Read the model definition and answer for the solid it produces. Units are mm, in the model's axes. A direction names the side the tool comes from. Give positions to 0.01 mm unless a question says otherwise; leave off trailing zeros. Order: outer loops, then holes, each group sorted by start corner. A loop starts at its lowest first (then second) coordinate and runs counter-clockwise, first axis right, second up. Notation, with made-up numbers: (-37.5, -8) -> (6.5, -8) arc R11 ccw to (6.5, -1) -> close; hole circle Ø1 at (-22.75, 8). An arc over 180 degrees is marked (long way). Answer as CSV lines item,"result". Start each with the question number.
1) For faces 1 (the face through (-3.905, 0.986, -0.867)), 2 (the face through (-10, 7, 13)), determine the directions among +Z, -Z, +X, -X, +Y, -Y from which every point of the face is accessible in a straight line to the end or side of a thin tool.
2) The mould has two halves that part along X. Classify faces 3 (the face through (0, 1, -12)), 4 (the face through (11, 15, 18)), 5 (the face through (2, 2, 4)), 6 (the face through (-12, 6, 12)): +X half, -X half, draft (parallel to the pull), parting line (faces both ways), or undercut.
3) Find section C-C (y = 13.75). Determine the outline of the cut face in (x, z), and give its area (3 significant figures).
4) Find section D-D (y = 1). Determine the outline of the cut face in (x, z).
5) Find section B-B (z = 16). Determine the outline of the cut face in (x, y).
6) Straight lines are drawn through the part: L1, parallel to X at y = 0.95, z = 0; L2, parallel to X at y = 4.5, z = 11; L3, parallel to Y at x = 9, z = 15. For each, find the intervals that lie inside material, in ascending order. Write a range as from..to.
7) Flat-ended cylindrical pins translate along their axes: pin 1 Ø2 at (x, z) = (0.5, 14) entering from -Y; pin 2 Ø2 at (x, z) = (6.5, 1.5) entering from +Y; pin 3 Ø4 at (y, z) = (3, -5.5) entering from +X. Find the tip coordinate at first contact, or state that the pin passes through.
8) Find section A-A (x = 0). Determine the outline of the cut face in (y, z), and give its area (3 significant figures).
```python
from build123d import *

# Parameters (mm, degrees)
SKETCH_1_R          = 12
SKETCH_1_R_2        = 4
EXTRUDE_1_DEPTH     = 2
EXTRUDE_2_DEPTH     = 2
BOSS_EXTRUDE1_START = -24
BOSS_EXTRUDE1_DEPTH = 2


with BuildPart() as part:
    # 草图1 → 凸台-拉伸1 (new body)
    # profile 1 of 2: a face of its own
    with BuildSketch(Plane(origin=(0, 0, 0), x_dir=(1, 0, 0), z_dir=(0, 1, 0))):
        Circle(SKETCH_1_R)
        with Locations(Location((0, 0, 0), (0, 0, 270))):
            Circle(SKETCH_1_R_2, mode=Mode.SUBTRACT)
    # profile 2 of 2: a face of its own
    with BuildSketch(Plane(origin=(0, 0, 0), x_dir=(1, 0, 0), z_dir=(0, 1, 0))):
        with BuildLine():
            ThreePointArc((12, 0), (0, -12), (-12, 0))
            Line((-12, 0), (-12, -20))
            Line((-12, -20), (12, -20))
            Line((12, -20), (12, 0))
        make_face()
    extrude(amount=EXTRUDE_1_DEPTH)

    # 草图3 → 凸台-拉伸2 (add)
    with BuildSketch(Plane(origin=(12, 0, 0), x_dir=(0, 0, -1), z_dir=(1, 0, 0))):
        Polygon((-20, 2), (-20, 15), (-15, 15), (-3, 2), align=None)
    extrude(amount=-EXTRUDE_2_DEPTH)

    # 草图3<2> → Boss-Extrude1 (add)
    with BuildSketch(Plane(origin=(12, 0, 0), x_dir=(0, 0, -1), z_dir=(1, 0, 0)).offset(BOSS_EXTRUDE1_START)):
        Polygon((-20, 2), (-20, 15), (-15, 15), (-3, 2), align=None)
    extrude(amount=BOSS_EXTRUDE1_DEPTH)


solid = part.part
```
Findings below:
1,face 1,"+Y, -Y"
1,face 2,"+Z, -Z, +Y"
2,face 3,"parting line"
2,face 4,"draft"
2,face 5,"undercut"
2,face 6,"-X half"
3,outline,"(-12, 13.85) -> (-10, 13.85) -> (-10, 20) -> (-12, 20) -> close; (10, 13.85) -> (12, 13.85) -> (12, 20) -> (10, 20) -> close"
3,area,"24.6 mm²"
4,outline,"(-12, 0) arc R12 ccw to (12, 0) -> (12, 20) -> (-12, 20) -> close; hole circle Ø8 at (0, 0)"
5,outline,"(-12, 0) -> (12, 0) -> (12, 15) -> (10, 15) -> (10, 2) -> (-10, 2) -> (-10, 15) -> (-12, 15) -> close"
6,L1,"-12..-4, 4..12"
6,L2,"-12..-10, 10..12"
6,L3,"0..2"
7,pin 1,"y = 0"
7,pin 2,"y = 2"
7,pin 3,"x = 11.39"
8,outline,"(0, -12) -> (2, -12) -> (2, -4) -> (0, -4) -> close; (0, 4) -> (2, 4) -> (2, 20) -> (0, 20) -> close"
8,area,"48.0 mm²"
